The model under review builds one solid part; all positions refer to its coordinate system, in mm. A direction names the side the tool comes from. Round coordinates to 2 decimals unless told otherwise and drop trailing zeros. Write each loop counter-clockwise with the first axis right and the second up, starting at its lowest first coordinate (ties: lowest second). Pieces come first, ordered by that corner, then holes. Notation, with made-up numbers: (58, 13) -> (96, 13) arc R21 ccw to (96, 38) -> close; hole circle Ø1 at (-9.5, -37). An arc over 180 degrees is marked (long way). Answer as a JSON object with one key per item and string values. Group by question number.
1) We need section D-D, the plane z = 6.75. Write out the cut boundary in (x, y).
2) To check wall thickness, follow probe 1 along Z at (x, y) = (-4.75, 1.25); probe 2 along Z at (x, y) = (-5.75, -2.5); probe 3 along X at (y, z) = (8.5, 2). State the ranges of each line that lie inside material, in increasing order. Write a range as [from, to].
3) We need section A-A, the plane y = 0. Write out the cut boundary in (x, z), then the cut area to 3 significant figures.
4) We need section C-C, the plane z = 2.5. Write out the cut boundary in (x, y), then the cut area to 3 significant figures.
5) Insertion check: pin 1 Ø3 at (x, z) = (-2, 3.5) entering from -Y; pin 2 Ø1.5 at (x, z) = (-7, 2) entering from +Y; pin 3 Ø2 at (x, z) = (-1.5, 1.5) entering from +Y. Each pin has a flat end and moves straight along its axis. Give the tip position at first contact, or say it passes through.
6) Machinability: for faces 1 (the flat face through (3, -4, 4)), 2 (the flat face through (0, 0, 0)), which of the approach directions +Z, -Z, +X, -X, +Y, -Y give a long, thin tool a straight path to every point of the face, cutting with its end or side? Answer none if there is none.
from build123d import *

# Parameters (mm, degrees)
F2_R     = 10.5
F2_R_2   = 6
F3_DEPTH = 3
F2_R_3   = 4.2
F4_DEPTH = 4
F5_DEPTH = 7
F6_SIZE  = 1


with BuildPart() as f3:
    # F2 (on Top) → F3 (new body)
    with BuildSketch(Plane.XY):
        Circle(F2_R)
        Circle(F2_R_2, mode=Mode.SUBTRACT)
    extrude(amount=F3_DEPTH)

    # F2 (on Top) → F4 (join)
    with BuildSketch(Plane.XY):
        Circle(F2_R_2)
        Circle(F2_R_3, mode=Mode.SUBTRACT)
    extrude(amount=F4_DEPTH)

    # F2 (on Top) → F5 (join)
    with BuildSketch(Plane.XY):
        Circle(F2_R_3)
    extrude(amount=F5_DEPTH)

    # F6
    f6_edges = [f3.edges().sort_by_distance(p)[0] for p in [
        (-10.5, 0, 0),
    ]]
    chamfer(f6_edges, length=F6_SIZE)


solid = f3.part
Here are the results:
{
 "1": {"outline": "circle Ø8.4 at (0, 0)"},
 "2": {"probe 1": "z = [0, 4]", "probe 2": "z = [0, 3]", "probe 3": "x = [-6.16, 6.16]"},
 "3": {"outline": "(-10.5, 1) -> (-9.5, 0) -> (9.5, 0) -> (10.5, 1) -> (10.5, 3) -> (6, 3) -> (6, 4) -> (4.2, 4) -> (4.2, 7) -> (-4.2, 7) -> (-4.2, 4) -> (-6, 4) -> (-6, 3) -> (-10.5, 3) -> close", "area": "99.2 mm^2"},
 "4": {"outline": "circle Ø21 at (0, 0)", "area": "346 mm^2"},
 "5": {"pin 1": "stops at y = -10.48", "pin 2": "stops at y = 8.44", "pin 3": "stops at y = 10.49"},
 "6": {"face 1": "+Z", "face 2": "-Z, +X, -X, +Y, -Y"}
}
